Verification items for the finished model (mm, model axes). A direction names the side the tool comes from. Give positions to 0.01 mm unless a question says otherwise; leave off trailing zeros. Loops run counter-clockwise (first coordinate to the right, second up) from the corner with the lowest first, then second, coordinate; pieces in that order, holes last. Notation, with made-up numbers: (-32.5, -19.75) - (-12.5, -19.75) arc R22 ccw to (-12.5, 14.25) - close; hole circle Ø9 at (22, 73.5). An arc over 180 degrees is marked (long way). One line per item, written item: value. Start each with the question number.
1. Scan lines: L1, parallel to Y at x = -59, z = 37; L2, parallel to X at y = 1, z = 36; L3, parallel to Z at x = -82.5, y = -22.5. Record each from-to range of solid material in increasing order. Write a range as [from, to].
2. Mould release check, pull along X, two halves, no side actions. Record for faces 1 (the flat face through (-61.176, -1, 25)), 2 (the flat face through (-85, -18.324, 25)), 3 (the cylindrical face through (-51.32, -9.39, 39.36)): pulls with the +X half, pulls with the -X half, needs draft (parallel to the pull), parting line crosses it, or undercut.
3. Sectioned sample at A-A (z = 11.5). Record the cut outline in (x, y), plus the area to 3 significant figures.
4. Sectioned sample at C-C (x = -86). Record the cut outline in (y, z).
5. Sectioned sample at D-D (z = 46). Record the cut outline in (x, y).
6. Access from +Z, -Z, +X, -X, +Y, -Y to the whole of each face (thin tool, end or side, straight path). Record for faces 4 (the cylindrical face through (-89.297, -17.31, 27.276)), 5 (the flat face through (-92, -16.324, 25)), 6 (the flat face through (-102.856, -26, 25)).
7. Sectioned sample at B-B (z = 23.5). Record the cut outline in (x, y), plus the area to 3 significant figures.
8. Gauge pin test, flat ends, axial feed: pin 1 (21 mm diameter, centred on x = -85, z = 36, fed in from +Y); pin 2 (2 mm diameter, centred on y = -8.74, z = 10.77, fed in from +X); pin 3 (4.5 mm diameter, centred on y = 5.64, z = 10.77, fed in from -X); pin 4 (8 mm diameter, centred on x = -80.71, z = 24.57, fed in from +Y). Record the tip position at first contact, or that the pin passes through.
from build123d import *

# Parameters (mm, degrees)
BOSS_EXTRUDE1_DEPTH = 50
SKETCH2_R           = 1.7
CUT_EXTRUDE2_DEPTH  = 75.542415548
SKETCH3_R           = 3
CUT_EXTRUDE3_DEPTH  = 119.507616013
SKETCH4_R           = 9
CUT_EXTRUDE4_DEPTH  = 2


with BuildPart() as part:
    # Sketch1 → Boss-Extrude1 (new body)
    with BuildSketch(Plane.XY):
        Polygon((-41.176470588, 14.736470588), (-41.176470588, -36.323529412), (-102.855877095, -36.323529412), (-102.855877095, -16.323529412), (-61.176470588, -16.323529412), (-61.176470588, 14.736470588), align=None)
    extrude(amount=BOSS_EXTRUDE1_DEPTH)

    # Sketch2 → Cut-Extrude2 (cut, through all)
    with BuildSketch(Plane.ZY.offset(61.176470588)):
        with Locations((10.768169464, 5.635466658)):
            Circle(SKETCH2_R)
        with Locations((37.786974644, 5.635466658)):
            Circle(SKETCH2_R)
        with Locations((10.768169464, -8.740849467)):
            Circle(SKETCH2_R)
        with Locations((37.786974644, -8.740849467)):
            Circle(SKETCH2_R)
    extrude(amount=-CUT_EXTRUDE2_DEPTH, mode=Mode.SUBTRACT)

    # Sketch3 → Cut-Extrude3 (cut, through all)
    with BuildSketch(Plane(origin=(0, -16.323529412, 0), x_dir=(1, 0, 0), z_dir=(0, 1, 0))):
        with Locations(Location((-80.712404336, -24.573120592, 0), (0, 0, 180))):
            Circle(SKETCH3_R)
    extrude(amount=-CUT_EXTRUDE3_DEPTH, mode=Mode.SUBTRACT)

    # Sketch4 → Cut-Extrude4 (cut)
    with BuildSketch(Plane(origin=(0, -16.323529412, 0), x_dir=(1, 0, 0), z_dir=(0, 1, 0))):
        with Locations(Location((-80.712404336, -24.573120592, 0), (0, 0, 180))):
            Circle(SKETCH4_R)
    extrude(amount=-CUT_EXTRUDE4_DEPTH, mode=Mode.SUBTRACT)


solid = part.part
Results are:
1. L1: y = [-36.32, -10.25], [-7.23, 4.13], [7.14, 14.74]
1. L2: x = [-61.18, -41.18]
1. L3: z = [0, 22.16], [26.98, 50]
2. face 1: pulls with the -X half
2. face 2: undercut
2. face 3: needs draft
3. outline: (-102.86, -36.32) - (-41.18, -36.32) - (-41.18, -10.28) - (-61.18, -10.28) - (-61.18, -16.32) - (-102.86, -16.32) - close; (-61.18, -7.21) - (-41.18, -7.21) - (-41.18, 4.1) - (-61.18, 4.1) - close; (-61.18, 7.17) - (-41.18, 7.17) - (-41.18, 14.74) - (-61.18, 14.74) - close
3. area: 1,730 mm^2
4. outline: (-36.32, 0) - (-16.32, 0) - (-16.32, 17.29) - (-18.32, 17.29) - (-18.32, 31.86) - (-16.32, 31.86) - (-16.32, 50) - (-36.32, 50) - close
5. outline: (-102.86, -36.32) - (-41.18, -36.32) - (-41.18, 14.74) - (-61.18, 14.74) - (-61.18, -16.32) - (-102.86, -16.32) - close
6. face 4: +Y
6. face 5: +Z, -Z, -X, +Y
6. face 6: +Z, -Z, -X, +Y, -Y
7. outline: (-102.86, -36.32) - (-83.51, -36.32) - (-83.51, -18.32) - (-89.65, -18.32) - (-89.65, -16.32) - (-102.86, -16.32) - close; (-77.91, -36.32) - (-41.18, -36.32) - (-41.18, 14.74) - (-61.18, 14.74) - (-61.18, -16.32) - (-71.78, -16.32) - (-71.78, -18.32) - (-77.91, -18.32) - close
7. area: 1,720 mm^2
8. pin 1: stops at y = -16.32
8. pin 2: passes through
8. pin 3: stops at x = -61.18
8. pin 4: stops at y = -18.32
